from build123d import *

# Parameters (mm, degrees)
F1_DEPTH = 18.034
F0_R     = 1.9939
F2_DEPTH = 2.54


# Not quite as in the source:
# - a feature names something its author has since deleted; it is built from what else it names


with BuildPart() as f1:
    # F0 (on Top) → F1 (new body)
    with BuildSketch(Plane.XY):
        with BuildLine():
            ThreePointArc((24.892, 0), (0, 24.892), (-24.892, 0))
            ThreePointArc((-24.892, 0), (0, -24.892), (24.892, 0))
        make_face()
    extrude(amount=F1_DEPTH)

    # F0 (on Top) → F2 (join)
    with BuildSketch(Plane.XY):
        with BuildLine():
            ThreePointArc((-37.084, 0), (0, -37.084), (37.084, 0))
            ThreePointArc((37.084, 0), (0, 37.084), (-37.084, 0))
        make_face()
        with Locations((15.494, -26.8363952125)):
            Circle(F0_R, mode=Mode.SUBTRACT)
        with BuildLine():
            ThreePointArc((-28.9941, 0), (-30.988, -1.9939), (-32.9819, 0))
            ThreePointArc((-32.9819, 0), (-30.988, 1.9939), (-28.9941, 0))
        make_face(mode=Mode.SUBTRACT)
        with BuildLine():
            ThreePointArc((24.892, 0), (0, -24.892), (-24.892, 0))
            ThreePointArc((-24.892, 0), (0, 24.892), (24.892, 0))
        make_face(mode=Mode.SUBTRACT)
        with Locations((15.494, 26.8363952125)):
            Circle(F0_R, mode=Mode.SUBTRACT)
    extrude(amount=F2_DEPTH)


solid = f1.part
Input: part model. Units: mm. Frame: model coordinates. A direction names the side the tool comes from. Round coordinates to 2 decimals unless told otherwise and drop trailing zeros. Loops run counter-clockwise (first coordinate to the right, second up) from the corner with the lowest first, then second, coordinate; pieces in that order, holes last. Notation, with made-up numbers: M 18.5,9 L 24.5,9 A23 cw 24.5,23 Z; hole C 86,32.5 d2. An arc over 180 degrees is marked long. Answer as CSV lines item,"result". Start each with the question number.
(1) Section D-D, the plane z = 5.5. Output: boundary loops of the cut face in (x, y).
(2) Draft query along X for faces 1 (the flat face through (0, 0, 18.034)), 2 (the cylindrical face through (-22.994, 9.534, 10.179)), 3 (the cylindrical face through (-32.83, -0.76, 1.25)). Return one class per face: released by +X, released by -X, zero draft, split by the parting line, or undercut.
(3) Section B-B, the plane x = 15.5. Output: boundary loops of the cut face in (y, z).
(4) Line query: line 1 (Y direction, x = 0, z = 12); line 2 (Z direction, x = -25, y = -26); line 3 (X direction, y = -1.5, z = 8.5). Output: solid intervals per line, ascending. Write a range as [from, to].
(5) Section C-C, the plane x = 0. Output: boundary loops of the cut face in (y, z), plus the area to 3 significant figures.
(6) First-contact query: pin 1 (4 mm diameter, centred on x = -23, z = 12, fed in from +Y); pin 2 (8 mm diameter, centred on x = 21.5, z = 11, fed in from +Y); pin 3 (5 mm diameter, centred on x = -22.5, z = 12.5, fed in from -Y). Flat tips, straight axial feed; report the tip coordinate or a pass-through.
(7) Reachability of faces 4 (the flat face through (8, -24, 2.54)), 5 (the flat face through (-1, 1, 0)) from +Z, -Z, +X, -X, +Y, -Y: full face, straight path, thin tool, end or side. Return the list, or none.
(8) Section A-A, the plane y = 0. Output: boundary loops of the cut face in (x, z), plus the area to 3 significant figures.
Values found:
1,outline,"C 0,0 d49.78"
2,face 1,"zero draft"
2,face 2,"split by the parting line"
2,face 3,"undercut"
3,outline,"M -33.69,0 L -28.83,0 L -28.83,2.54 L -33.69,2.54 Z; M -24.84,0 L 24.84,0 L 24.84,2.54 L 19.48,2.54 L 19.48,18.03 L -19.48,18.03 L -19.48,2.54 L -24.84,2.54 Z; M 28.83,0 L 33.69,0 L 33.69,2.54 L 28.83,2.54 Z"
4,line 1,"y = [-24.89, 24.89]"
4,line 2,"z = [0, 2.54]"
4,line 3,"x = [-24.85, 24.85]"
5,outline,"M -37.08,0 L 37.08,0 L 37.08,2.54 L 24.89,2.54 L 24.89,18.03 L -24.89,18.03 L -24.89,2.54 L -37.08,2.54 Z"
5,area,"960 mm²"
6,pin 1,"stops at y = 13.36"
6,pin 2,"stops at y = 17.7"
6,pin 3,"stops at y = -14.82"
7,face 4,"+Z"
7,face 5,"-Z, +X, -X, +Y, -Y"
8,outline,"M -37.08,0 L -32.98,0 L -32.98,2.54 L -37.08,2.54 Z; M -28.99,0 L 37.08,0 L 37.08,2.54 L 24.89,2.54 L 24.89,18.03 L -24.89,18.03 L -24.89,2.54 L -28.99,2.54 Z"
8,area,"950 mm²"
